CAD build for the part. Positions are in the model's coordinates, mm. A direction names the side the tool comes from. Coordinates: 2 decimals unless noted, no trailing zeros. Write each loop counter-clockwise with the first axis right and the second up, starting at its lowest first coordinate (ties: lowest second). Pieces come first, ordered by that corner, then holes. Notation, with made-up numbers: (49, -31) - (101, -31) arc R4 cw to (101, -27) - close; hole circle Ø11 at (34.25, -21). An arc over 180 degrees is marked (long way). Answer in a Markdown table with one row per item. Add a question column.
Q1. 3-axis set-ups, long thin cutter, end or side, ignore diameter. For faces 4 (the flat face through (0, 0, 34)), 5 (the cylindrical face through (0, -2, 18)), 6 (the flat face through (-0.15, 1.28, 0.89)): which of +Z, -Z, +X, -X, +Y, -Y reach the whole face in a straight line?
Q2. Two-plate mould, pull along X, no slides. Class faces 1 (the conical face through (0.47, 2.11, 2.44)), 2 (the flat face through (-1, -1.1, 0)), 3 (the flat face through (-1.033, -0.773, 0.887)): +X half, -X half, draft (parallel to the pull), parting line (faces both ways), or undercut.
Q3. Band-saw the part on A-A (x = 0). List the corners of the cut face in (y, z).
Q4. Band-saw the part on B-B (z = 19). List the corners of the cut face in (x, y).
Q5. Drill centre lines: line 1 along Z through (x, y) = (-0.25, -1); line 2 along Z through (x, y) = (1.25, -2.5); line 3 along Y through (x, z) = (-1.5, 20). Where is each one in solid material? Low to high. Write a range as from..to.
Q6. Pin check, flat tips, straight feed: pin 1 (1 mm diameter, centred on y = -1, z = 21.5, fed in from -X); pin 2 (5 mm diameter, centred on x = 3, y = -3.5, fed in from +Z); pin 3 (3 mm diameter, centred on y = 1, z = 5.5, fed in from -X). Stop position of each tip, or through.
```python
from build123d import *

# Parameters (mm, degrees)
SKETCH_1_R          = 2
EXTRUDE_1_DEPTH     = 34
CUT_EXTRUDE_1_DEPTH = 1.8


with BuildPart() as part:
    # 草图1 → 凸台-拉伸1 (new body)
    with BuildSketch(Plane.XY):
        Circle(SKETCH_1_R)
    extrude(amount=EXTRUDE_1_DEPTH)

    # 草图2 → 旋转1 (revolve)
    with BuildSketch(Plane(origin=(0, 0, 0), x_dir=(1, 0, 0), z_dir=(0, 1, 0)), mode=Mode.PRIVATE) as revolve_1_sk:
        Polygon((2, 0), (2, -2.6), (4.6, 0), align=None)
    revolve(revolve_1_sk.sketch.rotate(Axis((0, 0, 0), (0, 0, 1)), 180), axis=Axis((0, 0, 0), (0, 0, 1)))

    # 草图3 → 切除-拉伸1 (cut)
    with BuildSketch(Plane(origin=(0, 0, 0), x_dir=(-1, 0, 0), z_dir=(0, 0, -1))):
        Polygon((-0.59701127, 1.364689541), (-1.480361446, 0.165317844), (-0.883350176, -1.199371697), (0.59701127, -1.364689541), (1.480361446, -0.165317844), (0.883350176, 1.199371697), align=None)
    extrude(amount=-CUT_EXTRUDE_1_DEPTH, mode=Mode.SUBTRACT)


solid = part.part
```
Checked values:
| question | item | result |
|---|---|---|
| 1 | face 4 | +Z, +X, -X, +Y, -Y |
| 1 | face 5 | +Z |
| 1 | face 6 | -Z |
| 2 | face 1 | parting line |
| 2 | face 2 | draft |
| 2 | face 3 | undercut |
| 3 | outline | (-4.6, 0) - (-1.3, 0) - (-1.3, 1.8) - (1.3, 1.8) - (1.3, 0) - (4.6, 0) - (2, 2.6) - (2, 34) - (-2, 34) - (-2, 2.6) - close |
| 4 | outline | circle Ø4 at (0, 0) |
| 5 | line 1 | z = 1.8..34 |
| 5 | line 2 | z = 0..1.8 |
| 5 | line 3 | y = -1.32..1.32 |
| 6 | pin 1 | stops at x = -1.94 |
| 6 | pin 2 | stops at z = 2.49 |
| 6 | pin 3 | stops at x = -2 |
